```python
from build123d import *

# Parameters (mm, degrees)
BOSS_EXTRU_1_DEPTH = 8
ESQUISSE2_R        = 7.25
BOSS_EXTRU_2_DEPTH = 64
CONG_1_R           = 2


with BuildPart() as part:
    # Esquisse1 → Boss.-Extru.1 (new body)
    with BuildSketch(Plane(origin=(0, 0, 0), x_dir=(1, 0, 0), z_dir=(0, 1, 0))):
        Polygon((-10.392304845, 8.252712671), (-12.343211246, -4.873643664), (-1.950906401, -13.126356336), (10.392304845, -8.252712671), (12.343211246, 4.873643664), (1.950906401, 13.126356336), align=None)
    extrude(amount=BOSS_EXTRU_1_DEPTH)

    # Esquisse2 → Boss.-Extru.2 (add)
    with BuildSketch(Plane(origin=(0, 8, 0), x_dir=(1, 0, 0), z_dir=(0, 1, 0))):
        Circle(ESQUISSE2_R)
    extrude(amount=BOSS_EXTRU_2_DEPTH)

    # Congé1
    cong_1_edges = [part.edges().sort_by_distance(p)[0] for p in [
        (-7.25, 72, 0),
    ]]
    fillet(cong_1_edges, radius=CONG_1_R)


solid = part.part
```
Build history of the part. All positions in model axes, mm. A direction names the side the tool comes from. Coordinates: 2 decimals unless noted, no trailing zeros. Order: outer loops, then holes, each group sorted by start corner. A loop starts at its lowest first (then second) coordinate and runs counter-clockwise, first axis right, second up. Notation, with made-up numbers: (65.5, 35.25) -> (118.5, 35.25) arc R32 ccw to (118.5, 65.25) -> close; hole circle Ø10 at (87, 65). An arc over 180 degrees is marked (long way). Answer in a Markdown table with one row per item. Add a question column.
Q1. Band-saw the part on A-A, the plane x = 0. List the corners of the cut face in (y, z), then the cut area to 3 significant figures.
Q2. Band-saw the part on B-B, the plane y = 5.5. List the corners of the cut face in (x, z), then the cut area to 3 significant figures.
Q3. Band-saw the part on D-D, the plane z = 10.75. List the corners of the cut face in (x, y), then the cut area to 3 significant figures.
Q4. Drop flat-ended pins along their axis: pin 1 (6 mm diameter, centred on y = 18.5, z = -3, fed in from -X); pin 2 (3 mm diameter, centred on x = -6, y = 55, fed in from -Z); pin 3 (12 mm diameter, centred on y = 25, z = 3.5, fed in from +X); pin 4 (10 mm diameter, centred on x = 0.5, z = 8.5, fed in from -Y). Give the stop position or say it passes through.
Q5. Wall check: line 1 along X through (y, z) = (44.5, 0.25); line 2 along Y through (x, z) = (11.75, -2); line 3 along Z through (x, y) = (-5, 25.5). Give the ranges that are in metal, low to high. Write a range as [from, to].
Q6. Which spindle directions (+Z, -Z, +X, -X, +Y, -Y) get a long thin tool onto all of the face, cutting with end or side? Do faces 1 (the face through (3.35, 38.57, 6.43)), 2 (the face through (7.22, 3.94, -8.94)). Say none if no direction does.
Q7. Band-saw the part on C-C, the plane z = 0. List the corners of the cut face in (x, y).
Answers follow:
| question | item | result |
|---|---|---|
| 1 | outline | (0, -12.36) -> (8, -12.36) -> (8, -7.25) -> (70, -7.25) arc R2 ccw to (72, -5.25) -> (72, 5.25) arc R2 ccw to (70, 7.25) -> (8, 7.25) -> (8, 12.36) -> (0, 12.36) -> close |
| 1 | area | 1,120 mm^2 |
| 2 | outline | (-12.34, 4.87) -> (-10.39, -8.25) -> (1.95, -13.13) -> (12.34, -4.87) -> (10.39, 8.25) -> (-1.95, 13.13) -> close |
| 2 | area | 458 mm^2 |
| 3 | outline | (-4.94, 0) -> (4.07, 0) -> (4.07, 8) -> (-4.94, 8) -> close |
| 3 | area | 72.1 mm^2 |
| 4 | pin 1 | x = -7.25 |
| 4 | pin 2 | z = -5.68 |
| 4 | pin 3 | x = 7.25 |
| 4 | pin 4 | y = 0 |
| 5 | line 1 | [-7.25, 7.25] |
| 5 | line 2 | [0, 8] |
| 5 | line 3 | [-5.25, 5.25] |
| 6 | face 1 | +Y |
| 6 | face 2 | -Z, +X, +Y, -Y |
| 7 | outline | (-11.62, 0) -> (11.62, 0) -> (11.62, 8) -> (7.25, 8) -> (7.25, 70) arc R2 ccw to (5.25, 72) -> (-5.25, 72) arc R2 ccw to (-7.25, 70) -> (-7.25, 8) -> (-11.62, 8) -> close |
